The drawing under review shows one solid part. Ordinate dimensions are in mm from its lowest x, y, z. Round coordinates to 2 decimals unless told otherwise and drop trailing zeros. Loops run counter-clockwise (first coordinate to the right, second up) from the corner with the lowest first, then second, coordinate; pieces in that order, holes last. Notation, with made-up numbers: M 84,57.25 L 134,57.25 A14 cw 134,74.25 Z; hole C 7.5,82 d2. An arc over 180 degrees is marked long. Use a Markdown table: item, result.
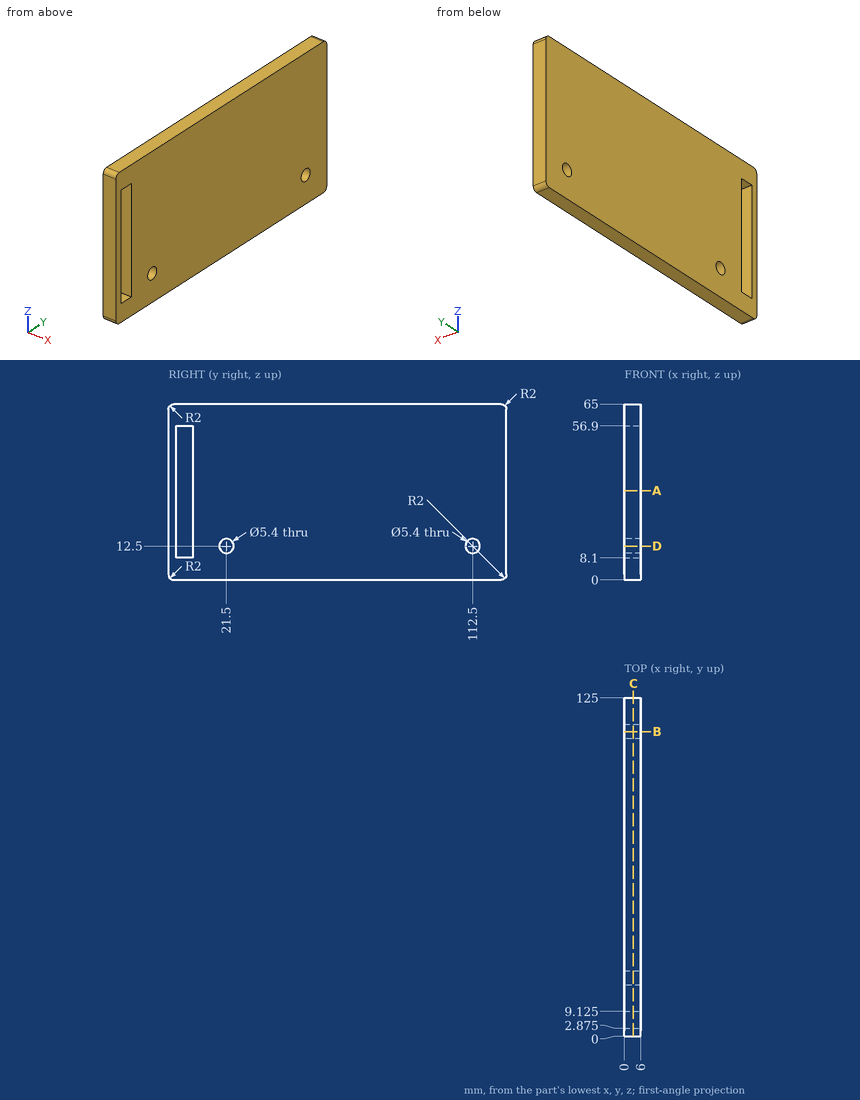
1. Take a section at B-B on y = 112.5. Give the boundary of the cut face in (x, z), and give its area (3 significant figures).
Check values:
| item | result |
|---|---|
| outline | M 0,0 L 6,0 L 6,9.8 L 0,9.8 Z; M 0,15.2 L 6,15.2 L 6,65 L 0,65 Z |
| area | 358 mm² |
2. Take a section at A-A on z = 33. Give the boundary of the cut face in (x, y) (3 decimals).
Check values:
| item | result |
|---|---|
| outline | M 0,0 L 6,0 L 6,2.875 L 0,2.875 Z; M 0,9.125 L 6,9.125 L 6,125 L 0,125 Z |
3. Take a section at D-D on z = 12.5. Give the boundary of the cut face in (x, y) (3 decimals).
Check values:
| item | result |
|---|---|
| outline | M 0,0 L 6,0 L 6,2.875 L 0,2.875 Z; M 0,9.125 L 6,9.125 L 6,18.8 L 0,18.8 Z; M 0,24.2 L 6,24.2 L 6,109.8 L 0,109.8 Z; M 0,115.2 L 6,115.2 L 6,125 L 0,125 Z |
4. Wall thickness on line 1 along Y through (x, z) = (5.05, 25.5) (3 decimals); line 2 along Z through (x, y) = (4.6, 21.5); line 3 along Y through (x, z) = (2.85, 13.5) (3 decimals): over which ranges is each line inside the solid? List them lowest first. Write a range as from..to.
Check values:
| item | result |
|---|---|
| line 1 | y = 0..2.875, 9.125..125 |
| line 2 | z = 0..9.8, 15.2..65 |
| line 3 | y = 0..2.875, 9.125..18.992, 24.008..109.992, 115.008..125 |
5. Take a section at C-C on x = 3.3. Give the boundary of the cut face in (y, z) (3 decimals), and give its area (3 significant figures).
Check values:
| item | result |
|---|---|
| outline | M 0,2 A2 ccw 2,0 L 123,0 A2 ccw 125,2 L 125,63 A2 ccw 123,65 L 2,65 A2 ccw 0,63 Z; hole M 2.875,8.1 L 9.125,8.1 L 9.125,56.9 L 2.875,56.9 Z; hole C 21.5,12.5 d5.4; hole C 112.5,12.5 d5.4 |
| area | 7,770 mm² |
